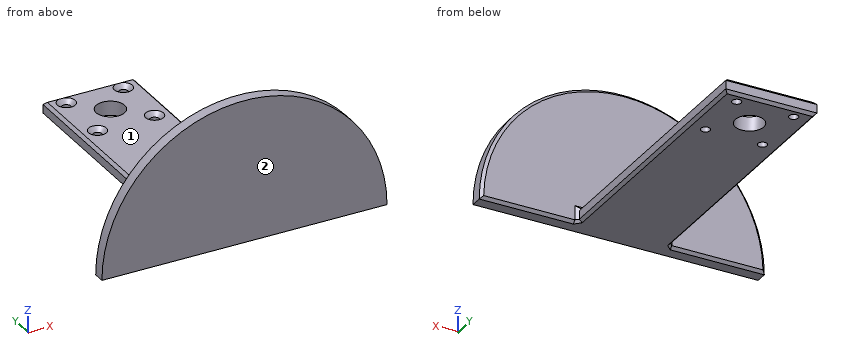
```python
from build123d import *

# Parameters (mm, degrees)
SKIZZE1_R                                            = 5
SKIZZE1_R_2                                          = 1.6
AUFSATZ_LINEAR_AUSTRAGEN1_DEPTH                      = 5
AUFSATZ_LINEAR_AUSTRAGEN2_DEPTH                      = 5
FASE1_SIZE                                           = 1
FASE2_SIZE                                           = 1
FASE3_SIZE                                           = 1
FORMSENKUNG_F_R_M3_LINSENSENKSCHRAUBE_MI_D           = 3.2
FORMSENKUNG_F_R_M3_LINSENSENKSCHRAUBE_MI_CSINK_D     = 6.3
FORMSENKUNG_F_R_M3_LINSENSENKSCHRAUBE_MI_CSINK_ANGLE = 90


with BuildPart() as part:
    # Skizze1 → Aufsatz-Linear austragen1 (new body)
    with BuildSketch(Plane.XY):
        Polygon((16, -13.386681205), (16, 7.597112796), (16, 14), (-16, 14), (-16, 4.559518535), (-16, -16.424275466), (-16, -86), (16, -86), align=None)
        Circle(SKIZZE1_R, mode=Mode.SUBTRACT)
        with Locations((10, -10)):
            Circle(SKIZZE1_R_2, mode=Mode.SUBTRACT)
        with Locations((-10, -10)):
            Circle(SKIZZE1_R_2, mode=Mode.SUBTRACT)
        with Locations((-10, 10)):
            Circle(SKIZZE1_R_2, mode=Mode.SUBTRACT)
        with Locations((10, 10)):
            Circle(SKIZZE1_R_2, mode=Mode.SUBTRACT)
    extrude(amount=AUFSATZ_LINEAR_AUSTRAGEN1_DEPTH)

    # Skizze2 → Aufsatz-Linear austragen2 (add)
    with BuildSketch(Plane(origin=(0, -86, 0), x_dir=(-1, 0, 0), z_dir=(0, -1, 0))):
        with BuildLine():
            Line((50, 0), (16, 0))
            Line((16, 0), (16, -5))
            Line((16, -5), (-16, -5))
            Line((-16, -5), (-16, 0))
            Line((-16, 0), (-50, 0))
            ThreePointArc((-50, 0), (0, -50), (50, 0))
        make_face()
    extrude(amount=-AUFSATZ_LINEAR_AUSTRAGEN2_DEPTH)

    # Fase1
    fase1_edges = [part.edges().sort_by_distance(p)[0] for p in [
        (16, -33.5, 0),
        (33, -81, 0),
        (-33, -81, 0),
        (0, -81, 50),
        (16, -81, 2.5),
        (0, -81, 5),
        (-16, -81, 2.5),
        (-16, -33.5, 0),
    ]]
    chamfer(fase1_edges, length=FASE1_SIZE)

    # Fase2
    fase2_edges = [part.edges().sort_by_distance(p)[0] for p in [
        (0, 14, 5),
        (-16, -33, 5),
        (16, -33, 5),
    ]]
    chamfer(fase2_edges, length=FASE2_SIZE)

    # Fase3
    fase3_edges = [part.edges().sort_by_distance(p)[0] for p in [
        (0, 14, 0),
    ]]
    chamfer(fase3_edges, length=FASE3_SIZE)

    # Formsenkung für M3 Linsensenkschraube mit Schlitz1 (through all)
    with Locations(Plane.XY.offset(5)):
        with Locations((-10, 10), (10, 10), (-10, -10), (10, -10)):
            CounterSinkHole(FORMSENKUNG_F_R_M3_LINSENSENKSCHRAUBE_MI_D / 2, FORMSENKUNG_F_R_M3_LINSENSENKSCHRAUBE_MI_CSINK_D / 2, counter_sink_angle=FORMSENKUNG_F_R_M3_LINSENSENKSCHRAUBE_MI_CSINK_ANGLE)


solid = part.part
```
For this review, take the finished solid that the model builds, in its own axes (mm). Face numbers are marked on the shaded views. A direction names the side the tool comes from. Give positions to 0.01 mm unless a question says otherwise; leave off trailing zeros. Loops run counter-clockwise (first coordinate to the right, second up) from the corner with the lowest first, then second, coordinate; pieces in that order, holes last. Notation, with made-up numbers: M 5.25,16 L 41.25,16 A19 cw 41.25,28 Z; hole C 70,6 d2. An arc over 180 degrees is marked long. One line per item, written item: value. Start each with the question number.
Q1. Add section C-C (y = -35.5). Give the boundary of the cut face in (x, z).
Q2. Add section A-A (x = 0). Give the boundary of the cut face in (y, z).
Q3. Clearance check with flat-ended pins moving along their axes: pin 1 Ø4 at (x, y) = (-10, 10) entering from -Z; pin 2 Ø12 at (x, z) = (-2, 18) entering from +Y; pin 3 Ø6 at (x, y) = (-18.5, -29.5) entering from +Z; pin 4 Ø0.9 at (y, z) = (-55, 2) entering from +X. State where each tip first meets the part, or that it passes through.
Q4. Machinability: for the marked faces 1 and 2, which of the approach directions +Z, -Z, +X, -X, +Y, -Y give a long, thin tool a straight path to every point of the face, cutting with its end or side? Answer none if there is none.
Q5. Add section B-B (y = 10). Give the boundary of the cut face in (x, z), and give its area (3 significant figures).
Q6. For L1, parallel to X at y = -10, z = 2; L2, parallel to Y at x = 10, z = 1.5; L3, parallel to Y at x = 0, z = 1.45, list the stretches that pass through material, from the lowest coordinate up.
Reply:
1. outline: M -16,1 L -15,0 L 15,0 L 16,1 L 16,4 L 15,5 L -15,5 L -16,4 Z
2. outline: M -86,0 L -5,0 L -5,5 L -80,5 L -81,6 L -81,49 L -82,50 L -86,50 Z; M 5,0 L 13,0 L 14,1 L 14,4 L 13,5 L 5,5 Z
3. pin 1: z = 0
3. pin 2: y = -81
3. pin 3: z = 4.5
3. pin 4: x = 16
4. face 1: +Z, +X, -X, +Y
4. face 2: +Z, -Z, +X, -X, -Y
5. outline: M -16,1 L -15,0 L -11.6,0 L -11.6,3.45 L -13.15,5 L -15,5 L -16,4 Z; M -8.4,0 L 8.4,0 L 8.4,3.45 L 6.85,5 L -6.85,5 L -8.4,3.45 Z; M 11.6,0 L 15,0 L 16,1 L 16,4 L 15,5 L 13.15,5 L 11.6,3.45 Z
5. area: 121 mm²
6. L1: -16 to -11.6, -8.4 to 8.4, 11.6 to 16
6. L2: -86 to -11.6, -8.4 to 8.4, 11.6 to 14
6. L3: -86 to -5, 5 to 14
